Could you check a few things on this model? Use its own coordinates, in mm. Give positions to 0.01 mm unless a question says otherwise; leave off trailing zeros. Write each loop counter-clockwise with the first axis right and the second up, starting at its lowest first coordinate (ties: lowest second). Pieces come first, ordered by that corner, then holes. Notation, with made-up numbers: M 23.5,-5 L 73.5,-5 A19 cw 73.5,31 Z; hole C 38.25,-32.5 d6. An arc over 180 degrees is marked long. Use one line per item in the form item = value.
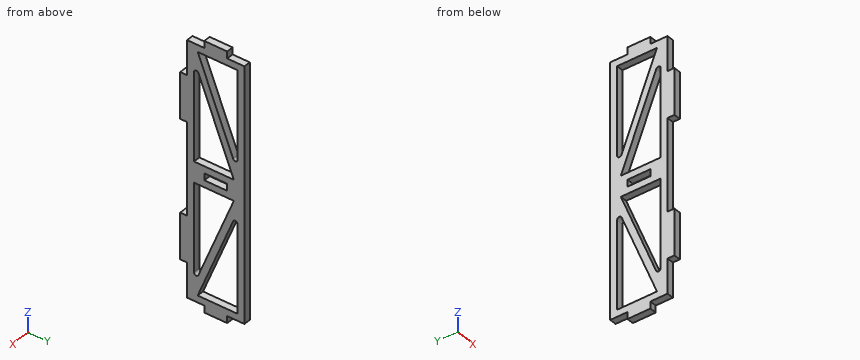
Autodesk Inventor part; units mm, degrees
ref_plane "YZ Plane" through (0, 0, 0) normal (1, 0, 0) x (0, 1, 0)
ref_plane "XZ Plane" through (0, 0, 0) normal (0, 1, 0) x (-1, 0, 0)
ref_plane "XY Plane" through (0, 0, 0) normal (0, 0, 1) x (1, 0, 0)
sketch "Sketch1" plane through (0, 0, 0) normal (1, 0, 0) x (0, 1, 0)
  line L0 (-12.5, -55) -> (12.5, -55)
  line L1 (12.5, -55) -> (12.5, 55)
  line L2 (12.5, 55) -> (-12.5, 55)
  line L3 (-12.5, 55) -> (-12.5, -55)
  line L4 (-12.5, -55) -> (12.5, 55) construction
  line L5 (12.5, -55) -> (-12.5, 55) construction
  point P0 (0, 0)
  dimension "d0" = 25
  dimension "d1" = 110
extrude "Extrusion1" add sketch "Sketch1" along normal blind 3
sketch "Sketch2" plane through (3, 0, 0) normal (1, 0, 0) x (0, 0, -1)
  line L0 (20, -12.5) -> (40, -12.5)
  line L1 (40, -12.5) -> (40, -15.5)
  line L2 (40, -15.5) -> (20, -15.5)
  line L3 (20, -15.5) -> (20, -12.5)
  line L4 (-55, -12.5) -> (55, -12.5)
  line L5 (-20, -12.5) -> (-40, -12.5)
  line L6 (-40, -12.5) -> (-40, -15.5)
  line L7 (-40, -15.5) -> (-20, -15.5)
  line L8 (-20, -15.5) -> (-20, -12.5)
  point P0 (0, 0)
  dimension "d4" = 20
  dimension "d5" = 3
  dimension "d6" = 20
  dimension "d7" = 20
  dimension "d8" = 3
  dimension "d9" = 20
extrude "Extrusion2" add sketch "Sketch2" against normal blind 3
sketch "Sketch3" plane through (3, 0, 0) normal (1, 0, 0) x (0, 0, -1)
  line L0 (-1.5, 5) -> (1.5, 5)
  line L1 (1.5, 5) -> (1.5, -5)
  line L2 (1.5, -5) -> (-1.5, -5)
  line L3 (-1.5, -5) -> (-1.5, 5)
  point P0 (0, 0)
  point P1 (-1.5, 0)
  point P2 (0, 5)
  dimension "d12" = 3
  dimension "d13" = 10
extrude "Extrusion3" cut sketch "Sketch3" against normal blind 3
sketch "Sketch4" plane through (3, 0, 0) normal (1, 0, 0) x (0, 0, -1)
  line L0 (55, -12.5) -> (55, 12.5)
  line L1 (55, 5) -> (58, 5)
  line L2 (58, 5) -> (58, -5)
  line L3 (58, -5) -> (55, -5)
  line L4 (55, -5) -> (55, 5)
  point P0 (0, 0)
  point P1 (58, 0)
  point P2 (55, 0)
  dimension "d16" = 3
  dimension "d17" = 10
extrude "Extrusion4" add sketch "Sketch4" against normal blind 3
sketch "Sketch5" plane through (3, 0, 0) normal (1, 0, 0) x (0, 0, -1)
  line L0 (4.5, 9.5) -> (52, 9.5)
  line L1 (52, 9.5) -> (52, -9.5)
  line L2 (52, -9.5) -> (4.5, -9.5)
  line L3 (4.5, -9.5) -> (4.5, 9.5)
  line L4 (55, 12.5) -> (-55, 12.5)
  line L5 (1.5, -5) -> (1.5, 5)
  line L6 (55, 5) -> (55, 12.5)
  line L7 (40, -12.5) -> (55, -12.5)
  point P0 (0, 0)
  dimension "d20" = 3
  dimension "d21" = 3
  dimension "d22" = 3
  dimension "d23" = 3
extrude "Extrusion5" cut sketch "Sketch5" against normal blind 3
sketch "Sketch6" plane through (3, 0, 0) normal (1, 0, 0) x (0, 0, -1)
  line L0 (4.5, 9.5) -> (52, -9.5) construction
  line L1 (3.9429, 8.1073) -> (51.4429, -10.8927)
  line L2 (52.5571, -8.1073) -> (5.0571, 10.8927)
  arc A0 (5.0571, 10.8927) -> (3.9429, 8.1073) centre (4.5, 9.5) ccw
  arc A1 (51.4429, -10.8927) -> (52.5571, -8.1073) centre (52, -9.5) ccw
  point P0 (0, 0)
  point P1 (28.25, 0)
  dimension "d26" = 3
extrude "Extrusion6" add sketch "Sketch6" against normal blind 3
fillet "Fillet1" radius 1 2 edges at (1.5, -9.5, -47.9611) (1.5, 9.5, -8.5389)
mirror "Mirror1" about plane through (0, 0, 0) normal (0, 0, 1) of "Extrusion5", "Extrusion6", "Fillet1", "Extrusion4"
equation "\"d23\" = d20"
properties part number "Battery holder"
1) For pin 1 Ø0.9 at (x, z) = (1.5, -56) entering from -Y; pin 2 Ø0.9 at (x, y) = (1, 9.5) entering from -Z; pin 3 Ø1.5 at (x, z) = (1, -5.5) entering from -Y, each with a flat end and sliding along its axis, tell me the tip position at first contact or that it passes through.
Checked values:
pin_1 = -5
pin_2 = -55
pin_3 = -12.5
2) I want a section at A-A, the plane z = -51. Please give me the cut outline in (x, y).
Checked values:
outline = M 0,-12.5 L 3,-12.5 L 3,-7.48 L 0,-7.48 Z; M 0,9.5 L 3,9.5 L 3,12.5 L 0,12.5 Z
3) I want a section at B-B, the plane y = 0. Please give me the cut outline in (x, z).
Checked values:
outline = M 0,-58 L 3,-58 L 3,-52 L 0,-52 Z; M 0,-32.29 L 3,-32.29 L 3,-24.21 L 0,-24.21 Z; M 0,-4.5 L 3,-4.5 L 3,-1.5 L 0,-1.5 Z; M 0,1.5 L 3,1.5 L 3,4.5 L 0,4.5 Z; M 0,24.21 L 3,24.21 L 3,32.29 L 0,32.29 Z; M 0,52 L 3,52 L 3,58 L 0,58 Z
4) If I drill on L1, parallel to Z at x = 2.1, y = -8.5; L2, parallel to Z at x = 2.85, y = 8.5; L3, parallel to Z at x = 1.25, y = -14, over which ranges is the centre line in solid material (lowest first)?
Checked values:
L1 = -55 to -43.77, -4.5 to 4.5, 43.77 to 55
L2 = -55 to -52, -12.73 to 12.73, 52 to 55
L3 = -40 to -20, 20 to 40
5) I want a section at C-C, the plane x = 1.3. Count the separate pieces of the cut face and the enclosed holes in it, plus the area to 3 significant figures.
Checked values:
separate_pieces = 1
enclosed_holes = 5
area = 1,400 mm2
6) I want a section at D-D, the plane z = 31. Please give me the cut outline in (x, y), plus the area to 3 significant figures.
Checked values:
outline = M 0,-15.5 L 3,-15.5 L 3,-9.5 L 0,-9.5 Z; M 0,-2.72 L 3,-2.72 L 3,0.52 L 0,0.52 Z; M 0,9.5 L 3,9.5 L 3,12.5 L 0,12.5 Z
area = 36.7 mm2
